```python
from build123d import *

# Parameters (mm, degrees)
SKETCH_1_W          = 60
SKETCH_1_H          = 70
SKETCH_1_R          = 28.65
EXTRUDE_1_DEPTH     = 30
SKETCH_2_W          = 76.072381137
SKETCH_2_H          = 88.67236145
CUT_EXTRUDE_1_DEPTH = 30
SKETCH_3_R          = 1.7
CUT_EXTRUDE_2_DEPTH = 40
SKETCH_4_W          = 20
SKETCH_4_H          = 14
CUT_EXTRUDE_3_DEPTH = 30
SKETCH_5_R          = 3.7
CUT_EXTRUDE_4_DEPTH = 10
FILLET_1_DEPTH      = 30


with BuildPart() as part:
    # 草图1 → 凸台-拉伸1 (new body)
    with BuildSketch(Plane(origin=(0, 0, 0), x_dir=(1, 0, 0), z_dir=(0, 1, 0))):
        Rectangle(SKETCH_1_W, SKETCH_1_H)
        with Locations(Location((0, 0, 0), (0, 0, 270))):
            Circle(SKETCH_1_R, mode=Mode.SUBTRACT)
    extrude(amount=EXTRUDE_1_DEPTH)

    # 草图2 → 切除-拉伸1 (cut)
    with BuildSketch(Plane(origin=(0, 30, 0), x_dir=(1, 0, 0), z_dir=(0, 1, 0))):
        with Locations((38.036190569, 1.889997047)):
            Rectangle(SKETCH_2_W, SKETCH_2_H)
    extrude(amount=-CUT_EXTRUDE_1_DEPTH, mode=Mode.SUBTRACT)

    # 草图3 → 切除-拉伸2 (cut)
    with BuildSketch(Plane(origin=(0, 0, 0), x_dir=(0, 0, -1), z_dir=(1, 0, 0))):
        with Locations((32, 20)):
            Circle(SKETCH_3_R)
        with Locations((-32, 20)):
            Circle(SKETCH_3_R)
    extrude(amount=-CUT_EXTRUDE_2_DEPTH, mode=Mode.SUBTRACT)

    # 草图4 → 切除-拉伸3 (cut)
    with BuildSketch(Plane(origin=(0, 0, -35), x_dir=(-1, 0, 0), z_dir=(0, 0, -1))):
        with Locations((20, 7)):
            Rectangle(SKETCH_4_W, SKETCH_4_H)
    extrude(amount=-CUT_EXTRUDE_3_DEPTH, mode=Mode.SUBTRACT)

    # 草图5 → 切除-拉伸4 (cut)
    with BuildSketch(Plane.ZY.offset(30)):
        with Locations((-32, 20)):
            Circle(SKETCH_5_R)
        with Locations((32, 20)):
            Circle(SKETCH_5_R)
    extrude(amount=-CUT_EXTRUDE_4_DEPTH, mode=Mode.SUBTRACT)

    # 圆角1: read off the stored shape, not the designer's step
    # 圆角1 outline → 圆角1 (cut)
    with BuildSketch(Plane(origin=(0, 0, 0), x_dir=(1, 0, 0), z_dir=(0, 1, 0))):
        with BuildLine():
            Line((-30, -35), (-20, -35))
            ThreePointArc((-20, -35), (-27.071067812, -32.071067812), (-30, -25))
            Line((-30, -25), (-30, -35))
        make_face()
        with BuildLine():
            Line((-30, 35), (-30, 25))
            ThreePointArc((-30, 25), (-27.071067812, 32.071067812), (-20, 35))
            Line((-20, 35), (-30, 35))
        make_face()
    extrude(amount=FILLET_1_DEPTH, mode=Mode.SUBTRACT)


solid = part.part
```
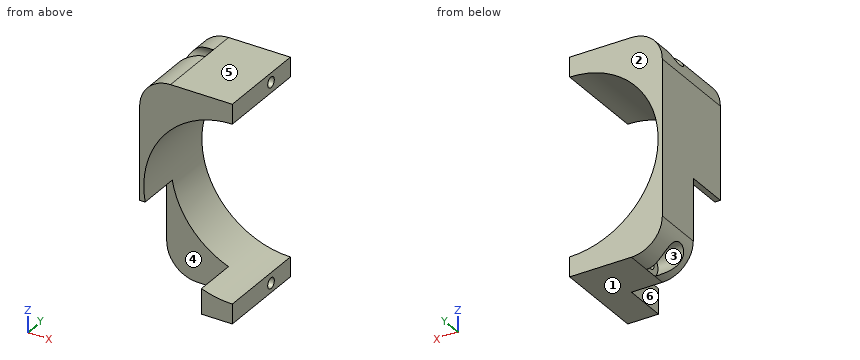
Input: part model. Units: mm. Frame: model coordinates. Face numbers are marked on the shaded views. A direction names the side the tool comes from. Coordinates: 2 decimals unless noted, no trailing zeros. Loops run counter-clockwise (first coordinate to the right, second up) from the corner with the lowest first, then second, coordinate; pieces in that order, holes last.
Q1. Mould query, pull axis Y, two halves, no side actions, for the marked faces 1, 2, 3 and 4. Classes: +Y half, -Y half, draft (parallel to the pull), parting line (faces both ways), or undercut.
Results are:
face 1: draft
face 2: +Y half
face 3: undercut
face 4: -Y half
Q2. Line query: line 1 along Y through (x, z) = (-11, -32); line 2 along Y through (x, z) = (-23, 32); line 3 along Y through (x, z) = (-19, -22.5). Output: solid intervals per line, ascending.
Results are:
line 1: y = 14 to 18.3, 21.7 to 30
line 2: y = 0 to 16.3, 23.7 to 30
line 3: y = 14 to 30
Q3. Set-up query: the marked faces 5 and 6. Return all of +Z, -Z, +X, -X, +Y, -Y with unobstructed straight access to the full face (end or side cutting, diameter ignored); none if empty.
Results are:
face 5: +Z, +X, -X, +Y, -Y
face 6: -Z, -X, -Y
Q4. Section C-C, the plane x = -16. Return the cut outline in (y, z).
Results are:
outline: (0, 23.77) - (30, 23.77) - (30, 35) - (0, 35) - close; (14, -35) - (30, -35) - (30, -23.77) - (14, -23.77) - close; hole circle Ø3.4 at (20, -32); hole circle Ø3.4 at (20, 32)
Q5. Contact query for flat-ended pins moving along their axis: pin 1 (1 mm diameter, centred on x = -21.5, y = 22.5, fed in from -Z); pin 2 (2 mm diameter, centred on y = 18, z = 31, fed in from -X); pin 3 (9.5 mm diameter, centred on y = 20, z = 32, fed in from -X); pin 4 (12 mm diameter, centred on x = -23.5, z = -6, fed in from -Y). Output: stop coordinate, or through.
Results are:
pin 1: stops at z = -34.95
pin 2: stops at x = -20
pin 3: stops at x = -29.74
pin 4: stops at y = 0
Q6. Section D-D, the plane z = -32. Return the cut outline in (x, y).
Results are:
outline: (-27.14, 14) - (-10, 14) - (-10, 0) - (0, 0) - (0, 18.3) - (-20, 18.3) - (-20, 16.3) - (-27.14, 16.3) - close; (-27.14, 23.7) - (-20, 23.7) - (-20, 21.7) - (0, 21.7) - (0, 30) - (-27.14, 30) - close
Q7. Section A-A, the plane y = 9. Return the cut outline in (x, z).
Results are:
outline: (-30, -5) - (-28.21, -5) arc R28.65 cw to (0, 28.65) - (0, 35) - (-20, 35) arc R10 ccw to (-30, 25) - close; (-10, -35) - (0, -35) - (0, -28.65) arc R28.65 cw to (-10, -26.85) - close
Q8. Section B-B, the plane y = 20. Return the cut outline in (x, z), and give its area (3 significant figures).
Results are:
outline: (-30, -25) arc R10 ccw to (-29.44, -28.3) - (-20, -28.3) - (-20, -30.3) - (0, -30.3) - (0, -28.65) arc R28.65 cw to (0, 28.65) - (0, 30.3) - (-20, 30.3) - (-20, 28.3) - (-29.44, 28.3) arc R10 ccw to (-30, 25) - close; (-20, -35) - (0, -35) - (0, -33.7) - (-20, -33.7) - close; (-20, 33.7) - (0, 33.7) - (0, 35) - (-20, 35) - close
area: 539 mm2
